```python
from build123d import *

# Parameters (mm, degrees)
SALIENTE_EXTRUIR1_DEPTH = 2.7


with BuildPart() as part:
    # Croquis1 → Saliente-Extruir1 (new body)
    with BuildSketch(Plane.YZ):
        with BuildLine():
            Line((69.812808286, -8.470319532), (69.813334046, -7.689593095))
            add(Edge.make_bspline(
                [(69.813334046, -7.689593095), (69.718277432, -7.690410058), (69.547216021, -7.691880338), (69.471672568, -7.54230989), (69.43809002, -7.475848405)],
                knots=[0, 0, 0, 0, 0.555650956, 1, 1, 1, 1], degree=3))
            add(Edge.make_bspline(
                [(69.43809002, -7.475848405), (69.485868998, -7.393671243), (69.571854074, -7.245781736), (69.739045293, -7.257082431), (69.813334046, -7.262103715)],
                knots=[0, 0, 0, 0, 0.555665944, 1, 1, 1, 1], degree=3))
            Line((69.813334046, -7.262103715), (69.813334046, -6.619874205))
            add(Edge.make_bspline(
                [(69.813334046, -6.619874205), (69.718281004, -6.62070628), (69.547206259, -6.62220393), (69.471672921, -6.472610717), (69.43809002, -6.406129515)],
                knots=[0, 0, 0, 0, 0.55558677, 1, 1, 1, 1], degree=3))
            add(Edge.make_bspline(
                [(69.43809002, -6.406129515), (69.485868647, -6.323952148), (69.571853089, -6.176062273), (69.739044357, -6.187362253), (69.813333131, -6.192383218)],
                knots=[0, 0, 0, 0, 0.555665944, 1, 1, 1, 1], degree=3))
            Line((69.813333131, -6.192383218), (69.812808286, -5.620390327))
            Line((69.812808286, -5.620390327), (65.824387706, -5.620390327))
            Line((65.824387706, -5.620390327), (65.823902281, -11.032305972))
            Line((65.823902281, -11.032305972), (39.747713095, -11.02806406))
            Line((39.747713095, -11.02806406), (39.748770289, -4.529207726))
            Line((39.748770289, -4.529207726), (36.898770326, -4.528744106))
            Line((36.898770326, -4.528744106), (36.897713133, -11.02760044))
            Line((36.897713133, -11.02760044), (20.486813862, -11.024930817))
            Line((20.486813862, -11.024930817), (20.487871055, -4.526074483))
            Line((20.487871055, -4.526074483), (17.637871093, -4.525610863))
            Line((17.637871093, -4.525610863), (17.636813899, -11.024467197))
            Line((17.636813899, -11.024467197), (1.226003887, -11.021797589))
            Line((1.226003887, -11.021797589), (1.22706108, -4.522941255))
            Line((1.22706108, -4.522941255), (-1.622938882, -4.522477635))
            Line((-1.622938882, -4.522477635), (-1.623996075, -11.021333969))
            Line((-1.623996075, -11.021333969), (-18.034716829, -11.018664376))
            Line((-18.034716829, -11.018664376), (-18.033659636, -4.519808041))
            Line((-18.033659636, -4.519808041), (-20.883659598, -4.519344421))
            Line((-20.883659598, -4.519344421), (-20.884716791, -11.018200756))
            Line((-20.884716791, -11.018200756), (-37.295526804, -11.015531148))
            Line((-37.295526804, -11.015531148), (-37.29446961, -4.516674813))
            Line((-37.29446961, -4.516674813), (-40.144469572, -4.516211193))
            Line((-40.144469572, -4.516211193), (-40.145526766, -11.015067527))
            Line((-40.145526766, -11.015067527), (-56.556426037, -11.012397905))
            Line((-56.556426037, -11.012397905), (-56.555368844, -4.51354157))
            Line((-56.555368844, -4.51354157), (-59.405368806, -4.51307795))
            Line((-59.405368806, -4.51307795), (-59.406426, -11.011934285))
            Line((-59.406426, -11.011934285), (-75.831996924, -11.009262276))
            Line((-75.831996924, -11.009262276), (-75.83152263, -4.510149615))
            Line((-75.83152263, -4.510149615), (-78.681522622, -4.509941627))
            Line((-78.681522622, -4.509941627), (-78.681996897, -11.008797361))
            Line((-78.681996897, -11.008797361), (-105.238788458, -11.008784177))
            add(Edge.make_bspline(
                [(-105.238788458, -11.008784177), (-105.14858271, -9.983450496), (-104.978798579, -8.052437708), (-103.415932971, -6.929206638), (-102.682870886, -6.402391424)],
                knots=[0, 0, 0, 0, 0.530982335, 1, 1, 1, 1], degree=3))
            add(Edge.make_bspline(
                [(-102.682870886, -6.402391424), (-101.394696585, -5.608529448), (-98.694632001, -3.944563162), (-93.215658737, -2.20965482), (-89.098251838, -1.412949472), (-86.602670214, -0.930072072)],
                knots=[0, 0, 0, 0, 0.264376639, 0.554143954, 1, 1, 1, 1], degree=3))
            add(Edge.make_bspline(
                [(-86.602670214, -0.930072072), (-84.973156703, -0.655698226), (-82.349752651, -0.213975311), (-79.694903541, -0.065172296), (-78.68908292, -0.008797357)],
                knots=[0, 0, 0, 0, 0.621144695, 1, 1, 1, 1], degree=3))
            Line((-78.68908292, -0.008797357), (58.126350502, -0.031053636))
            add(Edge.make_bspline(
                [(58.126350502, -0.031053636), (59.046945941, -0.03224198), (60.812517807, -0.034520976), (62.507529104, 0.456023838), (63.318712092, 0.690787646)],
                knots=[0, 0, 0, 0, 0.521422257, 1, 1, 1, 1], degree=3))
            add(Edge.make_bspline(
                [(63.318712092, 0.690787646), (65.143843319, 1.534523648), (69.06884794, 3.349005621), (75.404798534, 8.3094659), (79.947417099, 12.214266662), (82.743307297, 14.617606967)],
                knots=[0, 0, 0, 0, 0.250491315, 0.538689797, 1, 1, 1, 1], degree=3))
            add(Edge.make_bspline(
                [(82.743307297, 14.617606967), (85.047253105, 16.558828686), (88.71509394, 19.64921921), (92.441979531, 22.668023582), (93.827809061, 23.790572912)],
                knots=[0, 0, 0, 0, 0.628147706, 1, 1, 1, 1], degree=3))
            add(Edge.make_bspline(
                [(93.827809061, 23.790572912), (94.326453815, 24.199541627), (95.135569145, 24.863146035), (96.707492067, 25.728920147), (97.846009019, 25.692304846), (98.572307919, 25.668946364)],
                knots=[0, 0, 0, 0, 0.367687723, 0.596620683, 1, 1, 1, 1], degree=3))
            add(Edge.make_bspline(
                [(98.572307919, 25.668946364), (100.246973397, 25.678065075), (103.185898824, 25.694067802), (106.124806248, 25.676478931), (107.389032296, 25.668912593)],
                knots=[0, 0, 0, 0, 0.569822379, 1, 1, 1, 1], degree=3))
            add(Edge.make_bspline(
                [(107.389032296, 25.668912593), (108.060345413, 25.782878894), (108.783157194, 25.905587929), (109.548911413, 25.42625634), (109.482646974, 25.30201883), (109.444862485, 25.231273086)],
                knots=[0, 0, 0, 0, 0.848773339, 0.913885568, 1, 1, 1, 1], degree=3))
            add(Edge.make_bspline(
                [(109.444862485, 25.231273086), (109.370914057, 25.095380771), (109.105061218, 24.606832759), (108.522748832, 23.585003774), (107.54556697, 21.821989367), (106.764907477, 20.409086507), (106.284004774, 19.538728729)],
                knots=[0, 0, 0, 0, 0.071280186, 0.25626021, 0.541851204, 1, 1, 1, 1], degree=3))
            add(Edge.make_bspline(
                [(106.284004774, 19.538728729), (105.396909739, 17.909312095), (103.467658207, 14.365661847), (100.765990032, 9.360901344), (98.30554125, 4.781237125), (96.897745784, 2.110339814), (96.260543385, 0.901427017)],
                knots=[0, 0, 0, 0, 0.263007015, 0.571986842, 0.806270881, 1, 1, 1, 1], degree=3))
            add(Edge.make_bspline(
                [(96.260543385, 0.901427017), (95.874219388, 0.16818648), (95.240639904, -1.034343432), (94.500820955, -2.629812191), (93.945424943, -3.699029848), (93.988367719, -4.702342381), (93.914153339, -5.268329777), (93.868207957, -5.618726914)],
                knots=[0, 0, 0, 0, 0.352336975, 0.577840053, 0.756569684, 0.849294726, 1, 1, 1, 1], degree=3))
            Line((93.868207957, -5.618726914), (80.21346475, -5.623578454))
            Line((80.21346475, -5.623578454), (78.979630239, -5.623578454))
            Line((78.979630239, -5.623578454), (78.979601353, -6.200689117))
            add(Edge.make_bspline(
                [(78.979601353, -6.200689117), (79.074601125, -6.197779206), (79.245599405, -6.192542495), (79.324419315, -6.340422695), (79.359440945, -6.406129515)],
                knots=[0, 0, 0, 0, 0.555675338, 1, 1, 1, 1], degree=3))
            add(Edge.make_bspline(
                [(79.359440945, -6.406129515), (79.313479796, -6.48935539), (79.230789249, -6.639125118), (79.063383476, -6.631474374), (78.989003792, -6.628075089)],
                knots=[0, 0, 0, 0, 0.55569224, 1, 1, 1, 1], degree=3))
            Line((78.989003792, -6.628075089), (78.98995964, -7.269308448))
            add(Edge.make_bspline(
                [(78.98995964, -7.269308448), (79.085013314, -7.269607654), (79.256084268, -7.270146125), (79.329866383, -7.420596942), (79.36264575, -7.487448234)],
                knots=[0, 0, 0, 0, 0.555660155, 1, 1, 1, 1], degree=3))
            add(Edge.make_bspline(
                [(79.36264575, -7.487448234), (79.313911322, -7.569057991), (79.226204836, -7.715929624), (79.05916077, -7.702663194), (78.984935347, -7.696768304)],
                knots=[0, 0, 0, 0, 0.555653639, 1, 1, 1, 1], degree=3))
            Line((78.984935347, -7.696768304), (78.983701144, -8.470319532))
            Line((78.983701144, -8.470319532), (69.812808286, -8.470319532))
        make_face()
    extrude(amount=SALIENTE_EXTRUIR1_DEPTH)


solid = part.part
```
Could you check a few things on this model? Use its own coordinates, in mm. Coordinates: 2 decimals unless noted, no trailing zeros. Loops run counter-clockwise (first coordinate to the right, second up) from the corner with the lowest first, then second, coordinate; pieces in that order, holes last. Notation, with made-up numbers: M 8.25,-1 L 48.25,-1 A20 cw 48.25,34 Z; hole C 89,-20 d7. An arc over 180 degrees is marked long. Put each result on its own line as item: value. Start each with the question number.
(1) Will these pins go through, and if not, where does the flat tip stop? P1, Ø0.8, axis at x = 1, y = 38.5, coming from the -Z side; P2, Ø0.8, axis at x = 1, y = -65, coming from the -Z side; P3, Ø1.4, axis at x = 1, y = 75, coming from the -Z side.
(2) I need wall thicknesses on line 1 (Z direction, x = 0.95, y = 20); line 2 (Z direction, x = 0.6, y = -26.5); line 3 (Y direction, x = 2.1, z = 7.5). Which ranges of each line are inside material? Lowest first, please. Write a range as from..to.
(3) Suppose I cut it at A-A on y = 5. Please give me the cut outline in (x, z), then the cut area to 3 significant figures.
Solutions:
1. P1: stops at z = -4.53
1. P2: stops at z = -11.01
1. P3: stops at z = -8.47
2. line 1: z = -4.53..-0.02
2. line 2: z = -11.02..-0.02
2. line 3: y = 74.3..99.77
3. outline: M 0,-11.02 L 2.7,-11.02 L 2.7,-0.02 L 0,-0.02 Z
3. area: 29.7 mm2
